Drawing for the job (mm, zero at the part's lowest x, y, z). Coordinates: 2 decimals unless noted, no trailing zeros. Write each loop counter-clockwise with the first axis right and the second up, starting at its lowest first coordinate (ties: lowest second). Pieces come first, ordered by that corner, then holes. Notation, with made-up numbers: (73, -19.5) -> (89, -19.5) arc R8 ccw to (89, -5.5) -> close; hole circle Ø5 at (-3, 63). An arc over 180 degrees is marked (long way). Write item = value, one per line. Start each with the question number.
Q1. Band-saw the part on A-A, the plane y = 1.25. List the corners of the cut face in (x, z), plus the area to 3 significant figures.
Q2. Band-saw the part on B-B, the plane x = 20.5. List the corners of the cut face in (y, z), plus the area to 3 significant figures.
Q3. Band-saw the part on C-C, the plane x = 23.25. List the corners of the cut face in (y, z), plus the area to 3 significant figures.
Q4. Probe line 1 (Z direction, x = 8.25, y = 0.75); line 2 (Z direction, x = 3, y = 3.25); line 3 (X direction, y = 6.75, z = 46). List the from-to ranges inside material, lowest first.
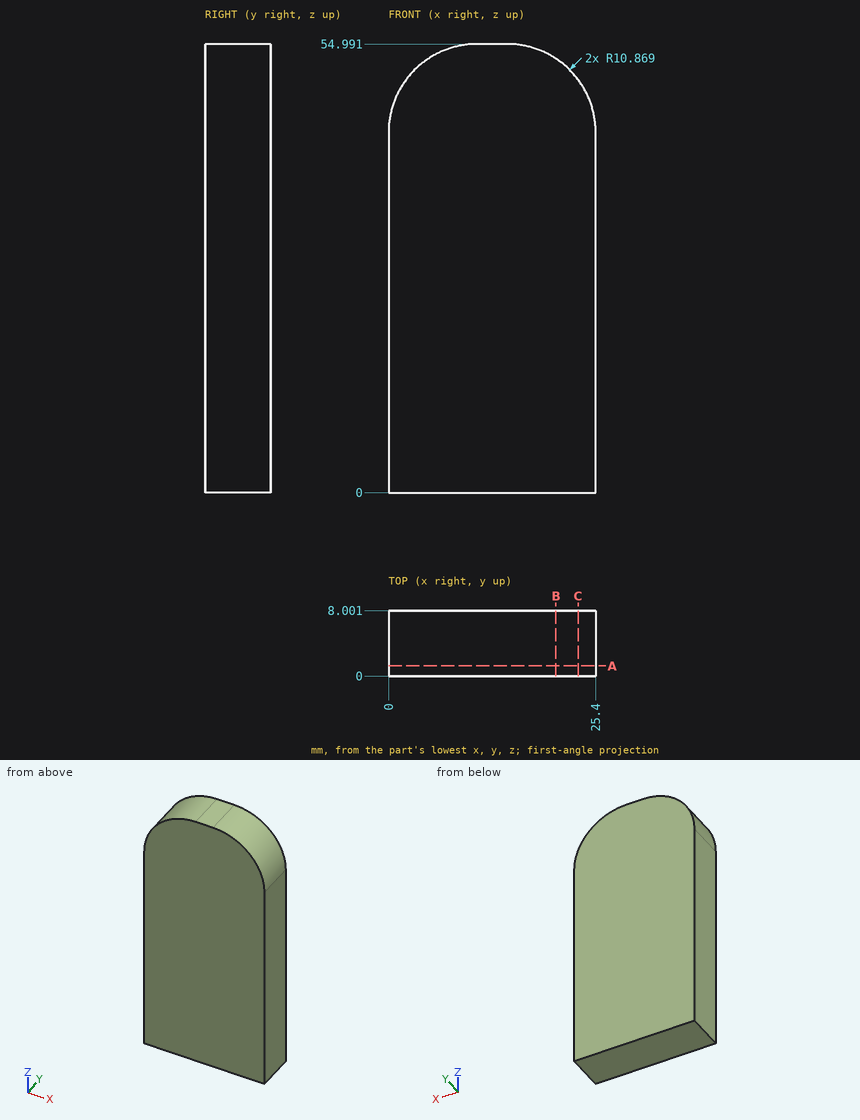
Ans:
q1.outline = (0, 0) -> (25.4, 0) -> (25.4, 44.12) arc R10.87 ccw to (14.53, 54.99) -> (10.87, 54.99) arc R10.87 ccw to (0, 44.12) -> close
q1.area = 1,350 mm2
q2.outline = (0, 0) -> (8, 0) -> (8, 53.21) -> (0, 53.21) -> close
q2.area = 426 mm2
q3.outline = (0, 0) -> (8, 0) -> (8, 50.61) -> (0, 50.61) -> close
q3.area = 405 mm2
q4.line_1 = 0 to 54.67
q4.line_2 = 0 to 51.62
q4.line_3 = 0.16 to 25.24
